```python
from build123d import *

# Parameters (mm, degrees)
SKETCH_1_W          = 68
SKETCH_1_H          = 44
EXTRUDE_1_DEPTH     = 2
FILLET_1_R          = 5.5
SKETCH_2_W          = 30
SKETCH_2_H          = 25
CUT_EXTRUDE_1_DEPTH = 3
FILLET_2_R          = 2
SKETCH_3_R          = 3
EXTRUDE_2_DEPTH     = 8.5
SKETCH_4_R          = 1.275
CUT_EXTRUDE_2_DEPTH = 6
CUT_EXTRUDE_2_TAPER = 2


with BuildPart() as part:
    # 草图1 → 凸台-拉伸1 (new body)
    with BuildSketch(Plane(origin=(0, 0, 0), x_dir=(1, 0, 0), z_dir=(0, 1, 0))):
        with Locations((-0.499435028, -2.675706215)):
            Rectangle(SKETCH_1_W, SKETCH_1_H)
    extrude(amount=EXTRUDE_1_DEPTH)

    # 圆角1
    fillet_1_edges = [part.edges().sort_by_distance(p)[0] for p in [
        (-34.499435028, 1, -19.324293785),
        (33.500564972, 1, -19.324293785),
        (33.500564972, 1, 24.675706215),
        (-34.499435028, 1, 24.675706215),
    ]]
    fillet(fillet_1_edges, radius=FILLET_1_R)

    # 草图2 → 切除-拉伸1 (cut, through all)
    with BuildSketch(Plane.XZ):
        with Locations((-0.499435028, 8.975706215)):
            Rectangle(SKETCH_2_W, SKETCH_2_H)
    extrude(amount=-CUT_EXTRUDE_1_DEPTH, mode=Mode.SUBTRACT)

    # 圆角2
    fillet_2_edges = [part.edges().sort_by_distance(p)[0] for p in [
        (14.500564972, 1, 21.475706215),
        (14.500564972, 1, -3.524293785),
        (-15.499435028, 1, -3.524293785),
        (-15.499435028, 1, 21.475706215),
    ]]
    fillet(fillet_2_edges, radius=FILLET_2_R)

    # 草图3 → 凸台-拉伸2 (add)
    with BuildSketch(Plane(origin=(0, 2, 0), x_dir=(1, 0, 0), z_dir=(0, 1, 0))):
        with Locations((-29.524435028, 2.549293785)):
            Circle(SKETCH_3_R)
        with Locations((-29.524435028, -20.500706215)):
            Circle(SKETCH_3_R)
        with Locations((28.500564972, -20.475706215)):
            Circle(SKETCH_3_R)
        with Locations((28.525564972, 2.549293785)):
            Circle(SKETCH_3_R)
    extrude(amount=EXTRUDE_2_DEPTH)

    # 草图4 → 切除-拉伸2 (cut)
    with BuildSketch(Plane(origin=(0, 10.5, 0), x_dir=(1, 0, 0), z_dir=(0, 1, 0))):
        with Locations((-29.524435028, 2.549293785)):
            Circle(SKETCH_4_R)
        with Locations((-29.499435028, -20.475706215)):
            Circle(SKETCH_4_R)
        with Locations((28.525564972, -20.500706215)):
            Circle(SKETCH_4_R)
        with Locations((28.525564972, 2.549293785)):
            Circle(SKETCH_4_R)
    extrude(amount=-CUT_EXTRUDE_2_DEPTH, taper=CUT_EXTRUDE_2_TAPER, mode=Mode.SUBTRACT)


solid = part.part
```
Source: CAD feature listing. Evaluate the final solid. Frame: model axes, mm. A direction names the side the tool comes from. Round coordinates to 2 decimals unless told otherwise and drop trailing zeros. Write each loop counter-clockwise with the first axis right and the second up, starting at its lowest first coordinate (ties: lowest second). Pieces come first, ordered by that corner, then holes. Notation, with made-up numbers: M -3,10.25 L 4,10.25 A18 cw 4,41.25 Z; hole C 56,-20 d3. An arc over 180 degrees is marked long. Use CSV: the item, a comma, the result in double quotes. Start each with the question number.
Q1. Access query for faces 1 (the face through (-30, 10.5, 22)), 2 (the face through (-1, 1, 21.476)), 3 (the face through (25.53, 6.19, -2.68)). Directions: +Z, -Z, +X, -X, +Y, -Y. A direction counts if a zero-diameter tool reaches every point of the face in a straight line with its end or side. Return the directions, or none.
Q2. Cut plane D-D on x = -21. Output: boundary loops of the cut face in (y, z).
Q3. Cut plane C-C on y = 8. Output: boundary loops of the cut face in (x, z), plus the area to 3 significant figures.
Q4. Line query: line 1 (Z direction, x = -6.5, y = 1); line 2 (Y direction, x = 22, z = 19.5); line 3 (Z direction, x = -31.5, y = 6). Output: solid intervals per line, ascending. Write a range as from..to.
Q5. Cut plane B-B on z = 15. Output: boundary loops of the cut face in (x, y), plus the area to 3 significant figures.
Q6. First-contact query: P1, Ø1.1, axis at x = 29, z = 20.5, coming from the +Y side; P2, Ø4, axis at y = 3.5, z = -8, coming from the -X side; P3, Ø1, axis at x = 17.5, z = 3, coming from the +Y side. Flat tips, straight axial feed; report the tip coordinate or a pass-through.
Q7. Pull-direction query (X, two-part tool) for faces 4 (the face through (31.847, 1.014, 23.107)), 5 (the face through (29, 10.5, 22)), 6 (the face through (-28.385, 7.458, 20.125)); classes: +X half, -X half, draft (parallel to the pull), parting line (faces both ways), or undercut.
Q8. Cut plane A-A on x = -5. Output: boundary loops of the cut face in (y, z), plus the area to 3 significant figures.
Results found:
1,face 1,"+Z, -Z, +X, -X, +Y"
1,face 2,"+Y, -Y"
1,face 3,"+Y"
2,outline,"M 0,-19.32 L 2,-19.32 L 2,24.68 L 0,24.68 Z"
3,outline,"C -29.52,-2.55 d6; C -29.52,20.5 d6; C 28.5,20.48 d6; C 28.53,-2.55 d6; hole C -29.52,-2.55 d2.38; hole C -29.5,20.48 d2.38; hole C 28.53,-2.55 d2.38; hole C 28.53,20.5 d2.38"
3,area,"95.4 mm^2"
4,line 1,"-19.32..-3.52, 21.48..24.68"
4,line 2,"0..2"
4,line 3,"-4.81..-0.29, 18.24..22.76"
5,outline,"M -34.5,0 L -15.5,0 L -15.5,2 L -34.5,2 Z; M 14.5,0 L 33.5,0 L 33.5,2 L 14.5,2 Z"
5,area,"76.0 mm^2"
6,P1,"y = 4.5"
6,P2,"x = -34.5"
6,P3,"y = 2"
7,face 4,"+X half"
7,face 5,"draft"
7,face 6,"undercut"
8,outline,"M 0,-19.32 L 2,-19.32 L 2,-3.52 L 0,-3.52 Z; M 0,21.48 L 2,21.48 L 2,24.68 L 0,24.68 Z"
8,area,"38.0 mm^2"
